Autodesk Inventor part; units mm, degrees
ref_plane "YZ Plane" through (0, 0, 0) normal (1, 0, 0) x (0, 1, 0)
ref_plane "XZ Plane" through (0, 0, 0) normal (0, 1, 0) x (-1, 0, 0)
ref_plane "XY Plane" through (0, 0, 0) normal (0, 0, 1) x (1, 0, 0)
sketch "Sketch1" plane through (0, 0, 0) normal (0, 1, 0) x (-1, 0, 0)
  line L0 (0, 0) -> (3.175, 0)
  line L1 (3.175, 0) -> (3.175, -6.35)
  line L2 (3.175, -6.35) -> (0, -6.35)
  line L3 (0, -6.35) -> (0, 0)
  line L4 (0, 0) -> (9.525, 0)
  line L5 (9.525, 0) -> (9.525, 8.255)
  line L6 (9.525, 8.255) -> (0, 8.255)
  line L7 (0, 8.255) -> (0, 0)
  line L8 (3.175, 0) -> (-6.35, 0)
  line L9 (-6.35, 0) -> (-6.35, 8.255)
  line L10 (-6.35, 8.255) -> (3.175, 8.255)
  line L11 (3.175, 8.255) -> (3.175, 0)
  dimension "d0" = 3.175
  dimension "d1" = 6.35
  dimension "d2" = 9.525
  dimension "d3" = 8.255
  dimension "d21" = 9.525
extrude "Extrusion1" add sketch "Sketch1" along normal blind 8.255 contours L7 L6 L11 L0 | L0 L1 L2 L3 | L8 L9 L10 L7
sketch "Sketch2" plane through (0, 0, 8.255) normal (1, 0, 0) x (0, 0, -1)
  line L0 (8.255, 8.255) -> (14.605, 8.255)
  line L1 (14.605, 8.255) -> (11.43, 8.255)
  line L2 (11.43, 8.255) -> (11.43, 5.08)
  line L3 (11.43, 5.08) -> (14.605, 5.08)
  line L4 (14.605, 5.08) -> (14.605, 8.255)
  point P0 (8.255, 0)
  point P1 (0, 8.255)
  dimension "d6" = 3.175
  dimension "d7" = 3.175
hole "Hole1" at (0, 5.08, -3.175) direction (-1, 0, 0) diameter 2.1565 depth 8.8646 tip angle 118
sketch "Sketch3" plane through (0, 8.255, 0) normal (0, 1, 0) x (1, 0, 0)
  line L0 (0, 0) -> (0, 6.35)
  line L1 (0, 6.35) -> (-3.175, 6.35)
  line L2 (-3.175, 6.35) -> (-3.175, -8.255)
  line L3 (-3.175, -8.255) -> (6.35, -8.255)
  line L4 (6.35, -8.255) -> (6.35, 0)
  line L5 (6.35, 0) -> (0, 0)
extrude "Extrusion2" cut sketch "Sketch3" against normal blind 0.75
sketch "Sketch4" plane through (0, 0, -6.35) normal (0, 0, -1) x (-1, 0, 0)
  line L0 (3.175, 7.505) -> (0, 7.505)
  line L1 (0, 0) -> (0, 7.505)
  line L2 (0, 0) -> (3.175, 0)
  line L3 (3.175, 0) -> (3.175, 7.505)
extrude "Extrusion3" cut sketch "Sketch4" against normal blind 0.75
sketch "Sketch5" plane through (-9.525, 0, 8.255) normal (0, 0, 1) x (1, 0, 0)
  line L0 (15.875, 7.505) -> (6.35, 7.505)
  line L1 (6.35, 0) -> (15.875, 0)
  line L2 (6.35, 0) -> (6.35, 7.505)
  line L3 (15.875, 0) -> (15.875, 7.505)
  line L4 (15.875, 7.505) -> (6.35, 7.505)
  line L5 (6.35, 0) -> (6.35, 7.505)
  line L6 (6.35, 0) -> (15.875, 0)
  line L7 (15.875, 0) -> (15.875, 7.505)
  point P0 (9.525, 0)
extrude "Extrusion4" cut sketch "Sketch5" against normal blind 0.75
sketch "Sketch6" plane through (6.35, 0, 0) normal (0, 0, -1) x (-1, 0, 0)
  line L0 (6.35, 7.505) -> (0, 7.505)
  line L1 (0, 0) -> (0, 7.505)
  line L2 (0, 0) -> (6.35, 0)
  line L3 (6.35, 0) -> (6.35, 7.505)
extrude "Extrusion5" cut sketch "Sketch6" against normal blind 0.75
fillet "Fillet1" radius 1.5875 3 edges at (1.5875, 7.505, 7.505) (-1.5875, 7.505, -5.6) (3.175, 7.505, 0.75)
fillet "Fillet2" radius 0.7937 1 edges at (6.35, 0, 4.1275)
properties part number "AFL-101-002-01-4E RetainerNut"
Input: part model. Units: mm. Frame: model coordinates. A direction names the side the tool comes from. Give positions to 0.01 mm unless a question says otherwise; leave off trailing zeros. Loops run counter-clockwise (first coordinate to the right, second up) from the corner with the lowest first, then second, coordinate; pieces in that order, holes last. Notation, with made-up numbers: M 35.5,37 L 50.5,37 A15 cw 50.5,45 Z; hole C 88,-1 d4. An arc over 180 degrees is marked long. Use CSV: the item, a comma, the result in double quotes.
(1) Pull-direction query (Z, two-part tool) for faces 3 (the face through (3.219, 7.028, 1.203)), 4 (the face through (1.52, 7.03, 7.05)), 5 (the face through (-1.6, 5, -2.1)); classes: pulls with the +Z half, pulls with the -Z half, needs draft (parallel to the pull), parting line crosses it, or undercut.
Outcome:
face 3,"pulls with the -Z half"
face 4,"pulls with the +Z half"
face 5,"undercut"
(2) Section A-A, the plane y = 5.08. Return loops of the section in (x, z) (3 decimals), plus the area to 3 significant figures.
Outcome:
outline,"M -3.175,-5.6 L 0,-5.6 L 0,-4.253 L -3.175,-4.253 Z; M -3.175,-2.097 L 0,-2.097 L 0,0.75 L 6.35,0.75 L 6.35,7.505 L -3.175,7.505 Z"
area,"77.7 mm²"
(3) Material intervals for L1, parallel to Z at x = -1.4, y = 5.08 (3 decimals); L2, parallel to X at y = 3.75, z = 0 (3 decimals); L3, parallel to Z at x = 2.5, y = 2.5 (3 decimals), sorted ascending. Write a range as [from, to].
Outcome:
L1,"z = [-5.6, -4.253], [-2.097, 7.505]"
L2,"x = [-3.175, 0]"
L3,"z = [0.75, 7.505]"
(4) Section C-C, the plane z = 1. Return loops of the section in (x, y) (3 decimals).
Outcome:
outline,"M -3.175,0 L 5.556,0 A0.794 ccw 6.35,0.794 L 6.35,6.773 L 0,6.773 L 0,7.505 L -3.175,7.505 Z"
(5) Pin query (flat end, axial travel): P1, Ø1.7, axis at y = 5.08, z = -3.175, coming from the -X side. Return the tip coordinate at first contact, or that it passes through.
Outcome:
P1,"passes through"
(6) Section D-D, the plane y = 1.25. Return loops of the section in (x, z) (3 decimals), plus the area to 3 significant figures.
Outcome:
outline,"M -3.175,-5.6 L 0,-5.6 L 0,0.75 L 6.35,0.75 L 6.35,7.505 L -3.175,7.505 Z"
area,"84.5 mm²"
(7) Set-up query: faces 1 (the face through (0, 0, 3)), 2 (the face through (3, 3, 0.75)). Return all of +Z, -Z, +X, -X, +Y, -Y with unobstructed straight access to the full face (end or side cutting, diameter ignored); none if empty.
Outcome:
face 1,"+Z, -Z, +X, -X, -Y"
face 2,"-Z, +X, +Y, -Y"
